Design review of the part shown in the three views and the two pictorial views. Dimensions are in mm from the part's minimum x, y and z. Round coordinates to 2 decimals unless told otherwise and drop trailing zeros. Write each loop counter-clockwise with the first axis right and the second up, starting at its lowest first coordinate (ties: lowest second). Pieces come first, ordered by that corner, then holes. Notation, with made-up numbers: (52.5, 5.25) -> (81.5, 5.25) arc R17 ccw to (81.5, 24.25) -> close; hole circle Ø10 at (40, -14.75). An arc over 180 degrees is marked (long way). Return JSON: item names as keys, results as strings. Group by question number.
1. Take a section at C-C, the plane z = 20. Write out the cut boundary in (x, y).
2. Take a section at D-D, the plane y = 7.5. Write out the cut boundary in (x, z).
3. Take a section at A-A, the plane x = 4.5. Write out the cut boundary in (y, z), then the cut area to 3 significant figures.
4. Clearance check with flat-ended pins moving along their axes: P1, Ø1.5, axis at y = 6.5, z = 9, coming from the +X side; P2, Ø3, axis at x = 1.5, z = 8.5, coming from the -Y side; P3, Ø1, axis at x = 3, z = 42, coming from the +Y side. State where each tip first meets the part, or that it passes through.
5. For line 1 along Z through (x, y) = (0.75, 3.75); line 2 along X through (y, z) = (4.75, 31), list the stretches that pass through material, from the lowest coordinate up. Write a range as from..to.
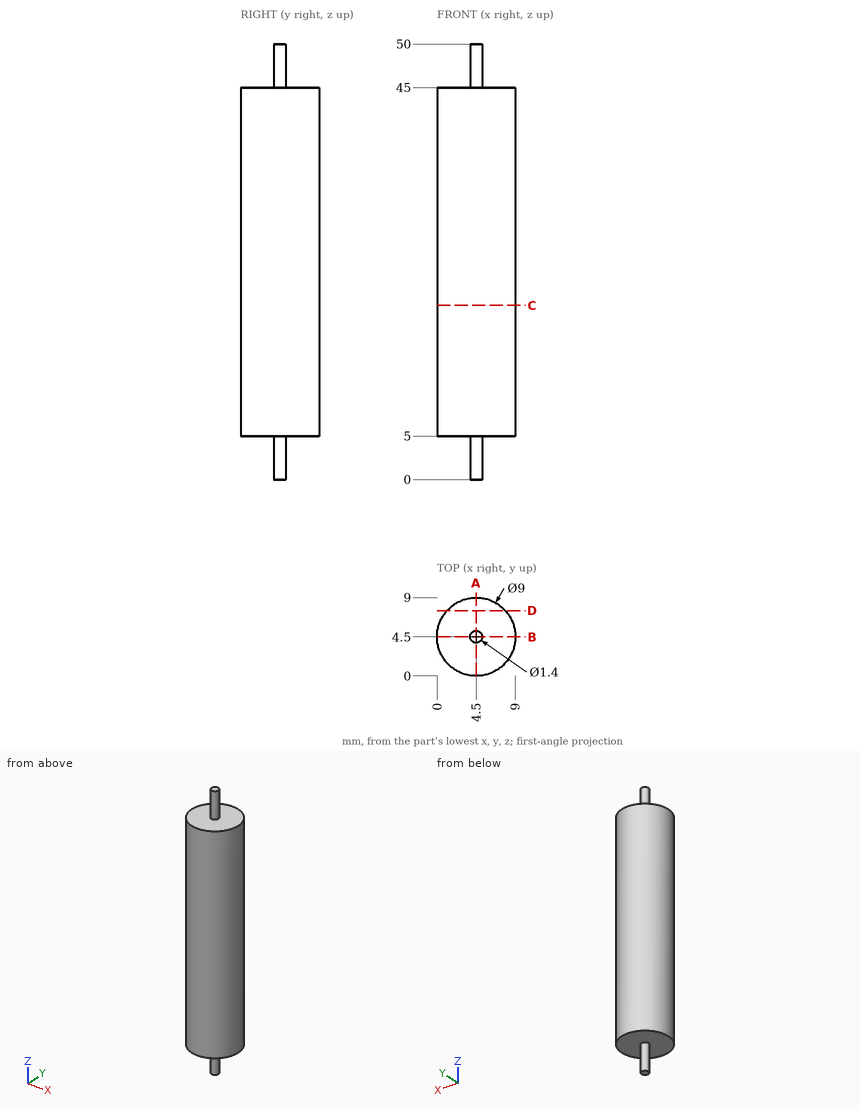
Output:
{
 "1": {"outline": "circle Ø9 at (4.5, 4.5)"},
 "2": {"outline": "(1.15, 5) -> (7.85, 5) -> (7.85, 45) -> (1.15, 45) -> close"},
 "3": {"outline": "(0, 5) -> (3.8, 5) -> (3.8, 0) -> (5.2, 0) -> (5.2, 5) -> (9, 5) -> (9, 45) -> (5.2, 45) -> (5.2, 50) -> (3.8, 50) -> (3.8, 45) -> (0, 45) -> close", "area": "374 mm^2"},
 "4": {"P1": "stops at x = 8.82", "P2": "stops at y = 0.26", "P3": "stops at y = 8.89"},
 "5": {"line 1": "z = 5..45", "line 2": "x = 0.01..8.99"}
}
